Read the model definition and answer for the solid it produces. Units are mm, in the model's axes. A direction names the side the tool comes from. Give positions to 0.01 mm unless a question says otherwise; leave off trailing zeros. Loops run counter-clockwise (first coordinate to the right, second up) from the corner with the lowest first, then second, coordinate; pieces in that order, holes last. Notation, with made-up numbers: M 6,10.5 L 49,10.5 A10 cw 49,24.5 Z; hole C 22,22 d2. An arc over 180 degrees is marked long. Return JSON: item names as keys, results as strings. Group by question number.
```python
from build123d import *

# Parameters (mm, degrees)
SKETCH1_W           = 67
SKETCH1_H           = 17
BOSS_EXTRUDE1_DEPTH = 53.5
FILLET1_R           = 2
FILLET2_R           = 8
SKETCH2_W           = 13
SKETCH2_H           = 6
CUT_EXTRUDE1_DEPTH  = 8


with BuildPart() as part:
    # Sketch1 → Boss-Extrude1 (new, symmetric)
    with BuildSketch(Plane(origin=(0, 0, 0), x_dir=(0, 0, -1), z_dir=(1, 0, 0))):
        with Locations((33.5, 8.5)):
            Rectangle(SKETCH1_W, SKETCH1_H)
    extrude(amount=BOSS_EXTRUDE1_DEPTH, both=True)

    # Fillet1
    fillet1_edges = [part.edges().sort_by_distance(p)[0] for p in [
        (53.5, 17, -33.5),
        (-53.5, 17, -33.5),
        (-53.5, 0, -33.5),
        (0, 17, 0),
        (0, 17, -67),
        (0, 0, -67),
        (0, 0, 0),
        (53.5, 0, -33.5),
    ]]
    fillet(fillet1_edges, radius=FILLET1_R)

    # Fillet2
    # the kernel refuses this fillet: 8 mm, written as the material it takes off along each edge
    with BuildSketch(Plane(origin=(45.5, 0, -8), x_dir=(1, 0, 0), z_dir=(0, 0, -1))) as fillet2_piece_1:
        with BuildLine():
            CenterArc((6, -2), 2, 0, 90)
            Line((8, -2), (8, 0))
            Line((8, 0), (6, 0))
        make_face()
    revolve(axis=Axis((45.5, 0, -8), (0, -1, 0)), revolution_arc=90, mode=Mode.SUBTRACT)
    with BuildSketch(Plane(origin=(45.5, 0, -59), x_dir=(0, 0, -1), z_dir=(-1, 0, 0))) as fillet2_piece_2:
        with BuildLine():
            CenterArc((6, -2), 2, 0, 90)
            Line((8, -2), (8, 0))
            Line((8, 0), (6, 0))
        make_face()
    revolve(axis=Axis((45.5, 0, -59), (0, -1, 0)), revolution_arc=90, mode=Mode.SUBTRACT)
    with BuildSketch(Plane(origin=(-45.5, 0, -8), x_dir=(0, 0, 1), z_dir=(1, 0, 0))) as fillet2_piece_3:
        with BuildLine():
            CenterArc((6, -2), 2, 0, 90)
            Line((8, -2), (8, 0))
            Line((8, 0), (6, 0))
        make_face()
    revolve(axis=Axis((-45.5, 0, -8), (0, -1, 0)), revolution_arc=90, mode=Mode.SUBTRACT)
    with BuildSketch(Plane(origin=(-45.5, 0, -59), x_dir=(-1, 0, 0), z_dir=(0, 0, 1))) as fillet2_piece_4:
        with BuildLine():
            CenterArc((6, -2), 2, 0, 90)
            Line((8, -2), (8, 0))
            Line((8, 0), (6, 0))
        make_face()
    revolve(axis=Axis((-45.5, 0, -59), (0, -1, 0)), revolution_arc=90, mode=Mode.SUBTRACT)
    with BuildSketch(Plane(origin=(45.5, 17, -59), x_dir=(1, 0, 0), z_dir=(0, 0, 1))) as fillet2_piece_5:
        with BuildLine():
            CenterArc((6, -2), 2, 0, 90)
            Line((8, -2), (8, 0))
            Line((8, 0), (6, 0))
        make_face()
    revolve(axis=Axis((45.5, 17, -59), (0, 1, 0)), revolution_arc=90, mode=Mode.SUBTRACT)
    with BuildSketch(Plane(origin=(45.5, 17, -8), x_dir=(0, 0, 1), z_dir=(-1, 0, 0))) as fillet2_piece_6:
        with BuildLine():
            CenterArc((6, -2), 2, 0, 90)
            Line((8, -2), (8, 0))
            Line((8, 0), (6, 0))
        make_face()
    revolve(axis=Axis((45.5, 17, -8), (0, 1, 0)), revolution_arc=90, mode=Mode.SUBTRACT)
    with BuildSketch(Plane(origin=(-45.5, 17, -59), x_dir=(0, 0, -1), z_dir=(1, 0, 0))) as fillet2_piece_7:
        with BuildLine():
            CenterArc((6, -2), 2, 0, 90)
            Line((8, -2), (8, 0))
            Line((8, 0), (6, 0))
        make_face()
    revolve(axis=Axis((-45.5, 17, -59), (0, 1, 0)), revolution_arc=90, mode=Mode.SUBTRACT)
    with BuildSketch(Plane(origin=(-45.5, 17, -8), x_dir=(-1, 0, 0), z_dir=(0, 0, -1))) as fillet2_piece_8:
        with BuildLine():
            CenterArc((6, -2), 2, 0, 90)
            Line((8, -2), (8, 0))
            Line((8, 0), (6, 0))
        make_face()
    revolve(axis=Axis((-45.5, 17, -8), (0, 1, 0)), revolution_arc=90, mode=Mode.SUBTRACT)
    with BuildSketch(Plane(origin=(-53.5, 17, 0), x_dir=(0, 0, -1), z_dir=(0, -1, 0)), Plane(origin=(-53.5, 0, -67), x_dir=(0, 0, 1), z_dir=(0, 1, 0)), Plane(origin=(53.5, 17, 0), x_dir=(-1, 0, 0), z_dir=(0, -1, 0)), Plane(origin=(53.5, 0, -67), x_dir=(-1, 0, 0), z_dir=(0, 1, 0))) as fillet2_piece_9:
        with BuildLine():
            CenterArc((FILLET2_R, FILLET2_R), FILLET2_R, 180, 90)
            Line((0, FILLET2_R), (0, 0))
            Line((0, 0), (FILLET2_R, 0))
        make_face()
    extrude(amount=17, mode=Mode.SUBTRACT)

    # Sketch2 → Cut-Extrude1 (cut)
    with BuildSketch(Plane(origin=(53.5, 0, 0), x_dir=(0, 0, -1), z_dir=(1, 0, 0))):
        with Locations((29.5, 9)):
            Rectangle(SKETCH2_W, SKETCH2_H)
    extrude(amount=-CUT_EXTRUDE1_DEPTH, mode=Mode.SUBTRACT)


solid = part.part
```
1. The mould has two halves that part along Z. Classify faces 3 (the flat face through (45.5, 9, -29)), 4 (the flat face through (1, 8, 0)), 5 (the cylindrical face through (-52.93, 0.6, -33.86)): +Z half, -Z half, draft (parallel to the pull), parting line (faces both ways), or undercut.
2. Flat-ended cylindrical pins translate along their axes: P1, Ø1.8, axis at x = 50.5, y = 10, coming from the +Z side; P2, Ø1.8, axis at y = 10, z = -30.5, coming from the +X side; P3, Ø1.8, axis at x = 49.5, y = 10, coming from the -Z side. Find the tip coordinate at first contact, or state that the pin passes through.
3. Find section A-A (z = -33.5). Write down the section's boundary in (x, y).
4. For faces 1 (the cylindrical face through (-51.094, 8.409, -64.719)), 2 (the flat face through (50, 9, -36)), determine the directions among +Z, -Z, +X, -X, +Y, -Y from which every point of the face is accessible in a straight line to the end or side of a thin tool.
5. Straight lines are drawn through the part: line 1 along X through (y, z) = (11.25, -25.5); line 2 along X through (y, z) = (9, -6). For each, find the intervals that lie inside material, in ascending order.
Result:
{
 "1": {"face 3": "undercut", "face 4": "+Z half", "face 5": "draft"},
 "2": {"P1": "stops at z = -1.13", "P2": "stops at x = 45.5", "P3": "stops at z = -66.37"},
 "3": {"outline": "M -53.5,2 A2 ccw -51.5,0 L 51.5,0 A2 ccw 53.5,2 L 53.5,6 L 45.5,6 L 45.5,12 L 53.5,12 L 53.5,15 A2 ccw 51.5,17 L -51.5,17 A2 ccw -53.5,15 Z"},
 "4": {"face 1": "-Z, -X, +Y, -Y", "face 2": "+X"},
 "5": {"line 1": "x = -53.5 to 45.5", "line 2": "x = -53.25 to 53.25"}
}
